```python
from build123d import *

# Parameters (mm, degrees)
F0_W     = 79.1909694672
F0_H     = 112.4388724566
F0_R     = 19.6004589853
F1_DEPTH = 21.209
F2_R     = 5.08
F3_SIZE  = 5.08
F4_R     = 5.08


# Not quite as in the source:
# - a feature names something its author has since deleted; it is built from what else it names


with BuildPart() as f1:
    # F0 (on Front) → F1 (new body, symmetric)
    with BuildSketch(Plane.XZ):
        with Locations((-183.0625087023, 9.1222152114)):
            Rectangle(F0_W, F0_H)
        with Locations((-187.305867672, 13.2941789925)):
            Circle(F0_R, mode=Mode.SUBTRACT)
    extrude(amount=F1_DEPTH, both=True)

    # F2
    f2_edges = [f1.edges().sort_by_distance(p)[0] for p in [
        (-183.062509, -21.209, 65.341651),
        (-222.657993, -21.209, 9.122215),
        (-183.062509, -21.209, -47.097221),
        (-143.467024, -21.209, 9.122215),
        (-206.906327, -21.209, 13.294179),
    ]]
    fillet(f2_edges, radius=F2_R)

    # F3
    f3_edges = [f1.edges().sort_by_distance(p)[0] for p in [
        (-183.062509, 21.209, 65.341651),
    ]]
    chamfer(f3_edges, length=F3_SIZE)

    # F4
    f4_edges = [f1.edges().sort_by_distance(p)[0] for p in [
        (-143.467024, 21.209, 6.582215),
    ]]
    fillet(f4_edges, radius=F4_R)


solid = f1.part
```
Can you work these out from the model? Positions are in its coordinate system, mm. Coordinates: 2 decimals unless noted, no trailing zeros. Loops run counter-clockwise (first coordinate to the right, second up) from the corner with the lowest first, then second, coordinate; pieces in that order, holes last. Notation, with made-up numbers: (-29, 25) - (16, 25) arc R27 ccw to (16, 58) - close; hole circle Ø1 at (-10, 16.25). An arc over 180 degrees is marked (long way). Use a Markdown table: item, result.
Item 1: I want a section at B-B on y = 8. Please give me the cut outline in (x, z), and give its area (3 significant figures).
Numbers:
| item | result |
|---|---|
| outline | (-222.66, -47.1) - (-143.47, -47.1) - (-143.47, 65.34) - (-222.66, 65.34) - close; hole circle Ø39.2 at (-187.31, 13.29) |
| area | 7,700 mm2 |
Item 2: We'd pull the mould along X, two halves only. Please class faces 1 (the face through (-144.995, 19.76, 9.909)), 2 (the face through (-222.658, 2, 8)), 3 (the face through (-206.887, 2.801, 14.156)), 4 (the face through (-184, 0, 65.342)): released by +X, released by -X, zero draft, split by the parting line, or undercut.
Numbers:
| item | result |
|---|---|
| face 1 | released by +X |
| face 2 | released by -X |
| face 3 | undercut |
| face 4 | zero draft |
Item 3: If I drill on probe 1 along Z at (x, y) = (-200, -3); probe 2 along Z at (x, y) = (-186, -17); probe 3 along X at (y, z) = (3.5, 10.5), over which ranges is the centre line in solid material (lowest first)? Write a range as from..to.
Numbers:
| item | result |
|---|---|
| probe 1 | z = -47.1..-1.64, 28.23..65.34 |
| probe 2 | z = -47.02..-6.34, 32.93..65.27 |
| probe 3 | x = -222.66..-206.71, -167.91..-143.47 |
Item 4: I want a section at A-A on y = -17.5. Please give me the cut outline in (x, z), and give its area (3 significant figures).
Numbers:
| item | result |
|---|---|
| outline | (-222.47, -46.91) - (-143.66, -46.91) - (-143.66, 65.15) - (-222.47, 65.15) - close; hole circle Ø39.58 at (-187.31, 13.29) |
| area | 7,600 mm2 |
